Work out the finished part from the listing and answer in its coordinate system (mm). A direction names the side the tool comes from. Round coordinates to 2 decimals unless told otherwise and drop trailing zeros. Loops run counter-clockwise (first coordinate to the right, second up) from the corner with the lowest first, then second, coordinate; pieces in that order, holes last. Notation, with made-up numbers: (-36.75, -32) - (9.25, -32) arc R19 cw to (9.25, -5) - close; hole circle Ø8 at (67.5, 12.5). An arc over 180 degrees is marked (long way). Answer as CSV lines item,"result". Start each with the question number.
```python
from build123d import *

# Parameters (mm, degrees)
SKETCH_1_W                   = 200
SKETCH_1_H                   = 53.2
SKETCH_1_R                   = 6.5
SKETCH_1_R_2                 = 2.025
EXTRUDE_1_DEPTH              = 2
SKETCH_2_R                   = 20
CUT_EXTRUDE_1_DEPTH          = 5
CUT_EXTRUDE_2_DEPTH          = 10
SKETCH_4_R                   = 1.1
CUT_EXTRUDE_3_DEPTH          = 10
SKETCH_5_W                   = 100
SKETCH_5_H                   = 13.4
SKETCH_5_R                   = 1.6
EXTRUDE_2_DEPTH              = 4
EXTRUDE_3_DEPTH              = 4
SKETCH_7_R                   = 1.1
SKETCH_7_R_2                 = 15
EXTRUDE_4_DEPTH              = 4
SKETCH_9_R                   = 1.1
CUT_EXTRUDE_4_DEPTH          = 10
SKETCH_11_R                  = 1.6
CUT_EXTRUDE_6_DEPTH          = 4
FILLET_1_R                   = 6
SKETCH_17_W                  = 12.3
SKETCH_17_H                  = 15.2
CUT_EXTRUDE_9_DEPTH          = 4
CUT_EXTRUDE_10_DEPTH         = 4
CUT_EXTRUDE_11_DEPTH         = 4
FILLET_2_R                   = 1.5
CUT_EXTRUDE_12_DEPTH         = 4
FILLET_3_R                   = 1.5
SKETCH_21_R                  = 1.55
CUT_EXTRUDE_13_DEPTH         = 10
FILLET_4_R                   = 2
HOLE_WIZARD_M3_1_D           = 3.4
HOLE_WIZARD_M3_1_CSINK_D     = 6.3
HOLE_WIZARD_M3_1_CSINK_ANGLE = 90


with BuildPart() as part:
    # 草图1 → 凸台-拉伸1 (new, symmetric)
    with BuildSketch(Plane.XY):
        with Locations((-75.7, 0)):
            Rectangle(SKETCH_1_W, SKETCH_1_H)
        Circle(SKETCH_1_R, mode=Mode.SUBTRACT)
        with Locations((20.3, 22.6)):
            Circle(SKETCH_1_R_2, mode=Mode.SUBTRACT)
        with Locations((20.3, 12.6)):
            Circle(SKETCH_1_R_2, mode=Mode.SUBTRACT)
        with Locations((20.3, -12.6)):
            Circle(SKETCH_1_R_2, mode=Mode.SUBTRACT)
        with Locations((20.3, -22.6)):
            Circle(SKETCH_1_R_2, mode=Mode.SUBTRACT)
    extrude(amount=EXTRUDE_1_DEPTH, both=True)

    # 草图2 → 切除-拉伸1 (cut)
    with BuildSketch(Plane.XY.offset(2)):
        with Locations((-148, 0)):
            Circle(SKETCH_2_R)
    extrude(amount=-CUT_EXTRUDE_1_DEPTH, mode=Mode.SUBTRACT)

    # 草图3 → 切除-拉伸2 (cut)
    with BuildSketch(Plane.XY.offset(2)):
        with BuildLine():
            Line((-136.21195189, -26.6), (-139.272801212, -12.199836119))
            ThreePointArc((-139.272801212, -12.199836119), (-152.260230171, -14.382296023), (-161.963751735, -5.47847036))
            Line((-161.963751735, -5.47847036), (-175.7, -19.214718626))
            Line((-175.7, -19.214718626), (-175.7, -26.6))
            Line((-175.7, -26.6), (-136.21195189, -26.6))
        make_face()
    extrude(amount=-CUT_EXTRUDE_2_DEPTH, mode=Mode.SUBTRACT)

    # 草图4 → 切除-拉伸3 (cut)
    with BuildSketch(Plane.XY.offset(2)):
        with Locations((-141, 23.478713764)):
            Circle(SKETCH_4_R)
        with Locations((-131.166837432, -17.801534708)):
            Circle(SKETCH_4_R)
        with Locations((-171.833162568, -5.677179055)):
            Circle(SKETCH_4_R)
    extrude(amount=-CUT_EXTRUDE_3_DEPTH, mode=Mode.SUBTRACT)

    # 草图5 → 凸台-拉伸2 (add)
    with BuildSketch(Plane.XY.offset(2)):
        with Locations((-125.7, 33.3)):
            Rectangle(SKETCH_5_W, SKETCH_5_H)
        with Locations((-170.7, 37)):
            Circle(SKETCH_5_R, mode=Mode.SUBTRACT)
        with Locations((-150.7, 37)):
            Circle(SKETCH_5_R, mode=Mode.SUBTRACT)
    extrude(amount=-EXTRUDE_2_DEPTH)

    # 草图6 → 凸台-拉伸3 (add)
    with BuildSketch(Plane.XY.offset(2)):
        Polygon((-175.7, 40), (-178.7, 40), (-178.7, -22.214718626), (-175.7, -19.214718626), align=None)
    extrude(amount=-EXTRUDE_3_DEPTH)

    # 草图7 → 凸台-拉伸4 (add)
    # profile 1 of 4: a face of its own
    with BuildSketch(Plane.XY.offset(2)):
        with Locations((-141, 23.478713764)):
            Circle(SKETCH_7_R)
    # profile 2 of 4: a face of its own
    with BuildSketch(Plane.XY.offset(2)):
        with Locations((-171.833162568, -5.677179055)):
            Circle(SKETCH_7_R)
    # profile 3 of 4: a face of its own
    with BuildSketch(Plane.XY.offset(2)):
        with Locations((-131.166837432, -17.801534708)):
            Circle(SKETCH_7_R)
    # profile 4 of 4: a face of its own
    with BuildSketch(Plane.XY.offset(2)):
        with BuildLine():
            Line((-136.21195189, -26.6), (-178.7, -26.6))
            Line((-178.7, -26.6), (-178.7, -22.214718626))
            Line((-178.7, -22.214718626), (-165.73337825, -9.248096876))
            ThreePointArc((-165.73337825, -9.248096876), (-142.319693106, 19.176394697), (-138.16441215, -17.414396677))
            Line((-138.16441215, -17.414396677), (-136.21195189, -26.6))
        make_face()
        with Locations((-148, 0)):
            Circle(SKETCH_7_R_2, mode=Mode.SUBTRACT)
    extrude(amount=-EXTRUDE_4_DEPTH)

    # 草图9 → 切除-拉伸4 (cut)
    with BuildSketch(Plane.XY.offset(2)):
        with Locations((-138.043830116, 16.182542484)):
            Circle(SKETCH_9_R)
        with Locations((-164.182542484, 9.956169884)):
            Circle(SKETCH_9_R)
        with Locations((-157.956169884, -16.182542484)):
            Circle(SKETCH_9_R)
        with Locations((-131.817457516, -9.956169884)):
            Circle(SKETCH_9_R)
    extrude(amount=-CUT_EXTRUDE_4_DEPTH, mode=Mode.SUBTRACT)

    # 草图11 → 切除-拉伸6 (cut)
    with BuildSketch(Plane.XY.offset(2)):
        with Locations((-166.7, 21.5)):
            Circle(SKETCH_11_R)
        with Locations((-80.7, 21.5)):
            Circle(SKETCH_11_R)
        with Locations((-166.7, -21.5)):
            Circle(SKETCH_11_R)
        with Locations((-80.7, -21.5)):
            Circle(SKETCH_11_R)
    extrude(amount=-CUT_EXTRUDE_6_DEPTH, mode=Mode.SUBTRACT)

    # 圆角1
    fillet_1_edges = [part.edges().sort_by_distance(p)[0] for p in [
        (-178.7, -26.6, 0),
        (-75.7, 40, 0),
        (-75.7, 26.6, 0),
    ]]
    fillet(fillet_1_edges, radius=FILLET_1_R)

    # 草图17 → 切除-拉伸9 (cut)
    with BuildSketch(Plane.XY.offset(2)):
        with Locations((18.15, 0)):
            Rectangle(SKETCH_17_W, SKETCH_17_H)
        with BuildLine():
            Line((15.3, -11.1), (5.748043145, -11.1))
            ThreePointArc((5.748043145, -11.1), (0, -12.5), (-5.748043145, -11.1))
            Line((-5.748043145, -11.1), (-9, -11.1))
            Line((-9, -11.1), (-9, -20.6))
            Line((-9, -20.6), (15.3, -20.6))
            Line((15.3, -20.6), (15.3, -11.1))
        make_face()
        with BuildLine():
            ThreePointArc((-5.748043145, 11.1), (0, 12.5), (5.748043145, 11.1))
            Line((5.748043145, 11.1), (15.3, 11.1))
            Line((15.3, 11.1), (15.3, 20.6))
            Line((15.3, 20.6), (-9, 20.6))
            Line((-9, 20.6), (-9, 11.1))
            Line((-9, 11.1), (-5.748043145, 11.1))
        make_face()
    extrude(amount=-CUT_EXTRUDE_9_DEPTH, mode=Mode.SUBTRACT)

    # 草图18 → 切除-拉伸10 (cut)
    with BuildSketch(Plane.XY.offset(2)):
        Polygon((-20.281777038, -20.6), (-74.7, 16.95495454), (-74.7, -20.6), align=None)
        Polygon((-15, 20.6), (-69.418222962, 20.6), (-15, -16.95495454), align=None)
    extrude(amount=-CUT_EXTRUDE_10_DEPTH, mode=Mode.SUBTRACT)

    # 草图19 → 切除-拉伸11 (cut)
    with BuildSketch(Plane.XY.offset(2)):
        with BuildLine():
            Line((-139.99687561, -20.6), (-94.394315744, -20.6))
            Line((-94.394315744, -20.6), (-128.107736542, -9.62849181))
            ThreePointArc((-128.107736542, -9.62849181), (-133.012282903, -16.241254145), (-139.99687561, -20.6))
        make_face()
        with BuildLine():
            Line((-126.250978368, -3.92301645), (-84.7, -17.445135792))
            Line((-84.7, -17.445135792), (-84.7, 28.638447058))
            Line((-84.7, 28.638447058), (-127.106066696, 7.200940987))
            ThreePointArc((-127.106066696, 7.200940987), (-126.203602063, 3.650621453), (-125.9, 0))
            ThreePointArc((-125.9, 0), (-125.987919475, -1.969342776), (-126.250978368, -3.92301645))
        make_face()
        with BuildLine():
            Line((-162.7, 32), (-162.7, 16.502121076))
            ThreePointArc((-162.7, 16.502121076), (-145.366842593, 21.942572367), (-129.81300787, 12.555608996))
            Line((-129.81300787, 12.555608996), (-91.349571914, 32))
            Line((-91.349571914, 32), (-162.7, 32))
        make_face()
    extrude(amount=-CUT_EXTRUDE_11_DEPTH, mode=Mode.SUBTRACT)

    # 圆角2
    fillet_2_edges = [part.edges().sort_by_distance(p)[0] for p in [
        (-5.748043145, -11.1, 0),
        (5.748043145, -11.1, 0),
        (15.3, -11.1, 0),
        (15.3, -20.6, 0),
        (-9, -20.6, 0),
        (-9, -11.1, 0),
        (5.748043145, 11.1, 0),
        (-5.748043145, 11.1, 0),
        (-9, 11.1, 0),
        (-9, 20.6, 0),
        (15.3, 20.6, 0),
        (15.3, 11.1, 0),
        (-69.418222962, 20.6, 0),
        (-15, 20.6, 0),
        (-15, -16.95495454, 0),
        (-20.281777038, -20.6, 0),
        (-74.7, -20.6, 0),
        (-74.7, 16.95495454, 0),
        (-126.250978368, -3.92301645, 0),
        (-127.106066696, 7.200940987, 0),
        (-84.7, 28.638447058, 0),
        (-84.7, -17.445135792, 0),
        (-129.81300787, 12.555608996, 0),
        (-162.7, 16.502121076, 0),
        (-162.7, 32, 0),
        (-91.349571914, 32, 0),
        (-139.99687561, -20.6, 0),
        (-128.107736542, -9.62849181, 0),
        (-94.394315744, -20.6, 0),
    ]]
    fillet(fillet_2_edges, radius=FILLET_2_R)

    # 草图20 → 切除-拉伸12 (cut)
    with BuildSketch(Plane.XY.offset(2)):
        with BuildLine():
            Line((-169.449244407, -17.998053071), (-164.469955527, -13.819933608))
            ThreePointArc((-164.469955527, -13.819933608), (-168.203391347, -7.353433082), (-169.5, 0))
            Line((-169.5, 0), (-176, 0))
            ThreePointArc((-176, 0), (-174.311393382, -9.576564013), (-169.449244407, -17.998053071))
        make_face()
        with BuildLine():
            ThreePointArc((-169.5, 0), (-168.767405265, 5.56460947), (-166.619546181, 10.75))
            Line((-166.619546181, 10.75), (-172.248711306, 14))
            ThreePointArc((-172.248711306, 14), (-175.045923136, 7.246933263), (-176, 0))
            Line((-176, 0), (-169.5, 0))
        make_face()
    extrude(amount=-CUT_EXTRUDE_12_DEPTH, mode=Mode.SUBTRACT)

    # 圆角3
    fillet_3_edges = [part.edges().sort_by_distance(p)[0] for p in [
        (-166.619546181, 10.75, 0),
        (-164.469955527, -13.819933608, 0),
        (-169.449244407, -17.998053071, 0),
        (-172.248711306, 14, 0),
    ]]
    fillet(fillet_3_edges, radius=FILLET_3_R)

    # 草图21 → 切除-拉伸13 (cut)
    with BuildSketch(Plane.XY.offset(2)):
        with Locations((-15, -22.6)):
            Circle(SKETCH_21_R)
    extrude(amount=-CUT_EXTRUDE_13_DEPTH, mode=Mode.SUBTRACT)

    # 圆角4
    fillet_4_edges = [part.edges().sort_by_distance(p)[0] for p in [
        (-178.7, 40, 0),
        (12, 7.6, 0),
        (24.3, 7.6, 0),
        (24.3, -7.6, 0),
        (12, -7.6, 0),
        (24.3, 26.6, 0),
        (24.3, -26.6, 0),
    ]]
    fillet(fillet_4_edges, radius=FILLET_4_R)

    # M3 锥坑平头螺钉的锥形沉头孔1 (through all)
    with Locations(Plane.XY.offset(2)):
        with Locations((-15, -22.6)):
            CounterSinkHole(HOLE_WIZARD_M3_1_D / 2, HOLE_WIZARD_M3_1_CSINK_D / 2, counter_sink_angle=HOLE_WIZARD_M3_1_CSINK_ANGLE)


solid = part.part
```
Item 1: Find the intervals of material crossed by L1, parallel to Y at x = -148, z = 0.3; L2, parallel to Y at x = -170.7, z = 0.4; L3, parallel to Y at x = -116, z = 0.2, in increasing order.
Item 2: Which of the six approach directions +Z, -Z, +X, -X, +Y, -Y give full straight-line access (tool end or side, diameter ignored) to faces 4 (the face through (-129, 32, 0)), 5 (the face through (-176.989, -24.796, -0.028))?
Item 3: Flat-ended cylindrical pins translate along their axes: pin 1 Ø1.9 at (x, y) = (-80.7, -21.5) entering from +Z; pin 2 Ø1.5 at (y, z) = (33, -0.5) entering from +X. Find the tip coordinate at first contact, or state that the pin passes through.
Item 4: Section B-B, the plane x = 20.3 is taken. Give the vertices of the cut face in (y, z) (3 decimals), and give its area (3 significant figures).
Item 5: Section A-A, the plane x = 0 is taken. Give the vertices of the cut face in (y, z), and give its area (3 significant figures).
Item 6: Section C-C, the plane z = 1.15 is taken. Count the separate pieces of the cut face and the enclosed holes in it, and give its area (3 significant figures).
Item 7: Determine the mould class of faces 1 (the face through (-79, 7, -2)), 2 (the face through (15.3, -16, 0)), 3 (the face through (-24, 26.6, 0)) for opening direction Y: pulls with the +Y half, pulls with the -Y half, needs draft (parallel to the pull), parting line crosses it, or undercut.
Answer:
1,L1,"y = -26.6 to -15, 15 to 22.1, 32 to 40"
1,L2,"y = -26.6 to -16.39, 13.11 to 35.4, 38.6 to 40"
1,L3,"y = -26.6 to -20.6, -13.57 to -7.26, 12.82 to 19.54, 32 to 40"
2,face 4,"+Z, -Z"
2,face 5,"+Z, -Z, -X, -Y"
3,pin 1,"passes through"
3,pin 2,"stops at x = -75.69"
4,outline,"(-26.6, -2) - (-24.625, -2) - (-24.625, 2) - (-26.6, 2) - close; (-20.575, -2) - (-14.625, -2) - (-14.625, 2) - (-20.575, 2) - close; (-10.575, -2) - (-7.6, -2) - (-7.6, 2) - (-10.575, 2) - close; (7.6, -2) - (10.575, -2) - (10.575, 2) - (7.6, 2) - close; (14.625, -2) - (20.575, -2) - (20.575, 2) - (14.625, 2) - close; (24.625, -2) - (26.6, -2) - (26.6, 2) - (24.625, 2) - close"
4,area,"87.2 mm²"
5,outline,"(-26.6, -2) - (-20.6, -2) - (-20.6, 2) - (-26.6, 2) - close; (-12.5, -2) - (-6.5, -2) - (-6.5, 2) - (-12.5, 2) - close; (6.5, -2) - (12.5, -2) - (12.5, 2) - (6.5, 2) - close; (20.6, -2) - (26.6, -2) - (26.6, 2) - (20.6, 2) - close"
5,area,"96.0 mm²"
6,separate pieces,"1"
6,enclosed holes,"25"
6,area,"6,170 mm²"
7,face 1,"needs draft"
7,face 2,"undercut"
7,face 3,"pulls with the +Y half"
